Answer from the drawing. Dimensions are ordinates in mm from the lowest x, y and z of the part. Coordinates: 2 decimals unless noted, no trailing zeros. Write each loop counter-clockwise with the first axis right and the second up, starting at its lowest first coordinate (ties: lowest second). Pieces come first, ordered by that corner, then holes.
(1) The part is cut by section B-B on x = 170.5. Determine the outline of the cut face in (y, z), plus the area to 3 significant figures.
(2) The part is cut by section A-A on z = 641. Determine the outline of the cut face in (x, y).
(3) The part is cut by section C-C on x = 481. Determine the outline of the cut face in (y, z).
(4) Straight lines are drawn through the part: line 1 (Z direction, x = 185, y = 15.25); line 2 (Z direction, x = 352.5, y = 16.75); line 3 (X direction, y = 9.25, z = 678.5). For each, find the intervals that lie inside material, in ascending order.
(5) The part is cut by section D-D on y = 7.75. Determine the outline of the cut face in (x, z).
(6) Given P1, Ø5.5, axis at x = 144.5, y = 10, coming from the -Z side, flat-ended and moving along its own axis, determine where the tip first touches the part or whether it passes through.
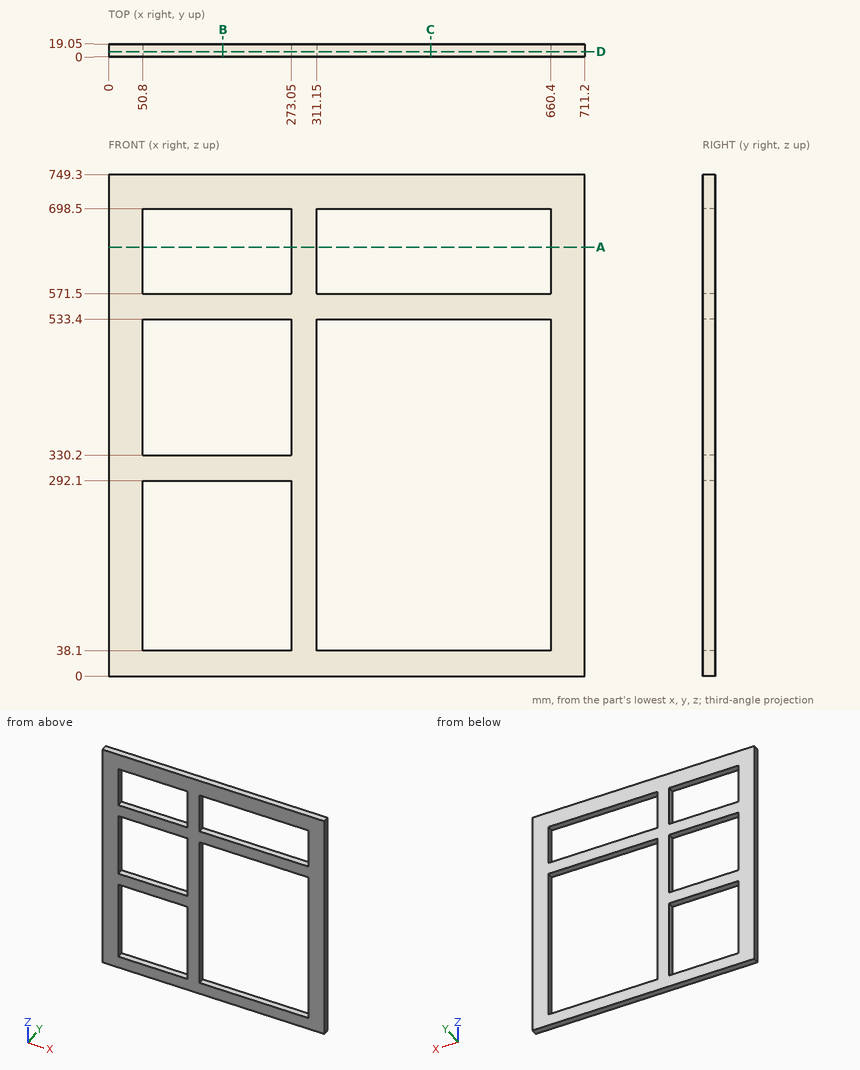
Model answer:
1. outline: (0, 0) - (19.05, 0) - (19.05, 38.1) - (0, 38.1) - close; (0, 292.1) - (19.05, 292.1) - (19.05, 330.2) - (0, 330.2) - close; (0, 533.4) - (19.05, 533.4) - (19.05, 571.5) - (0, 571.5) - close; (0, 698.5) - (19.05, 698.5) - (19.05, 749.3) - (0, 749.3) - close
1. area: 3,150 mm2
2. outline: (0, 0) - (50.8, 0) - (50.8, 19.05) - (0, 19.05) - close; (273.05, 0) - (311.15, 0) - (311.15, 19.05) - (273.05, 19.05) - close; (660.4, 0) - (711.2, 0) - (711.2, 19.05) - (660.4, 19.05) - close
3. outline: (0, 0) - (19.05, 0) - (19.05, 38.1) - (0, 38.1) - close; (0, 533.4) - (19.05, 533.4) - (19.05, 571.5) - (0, 571.5) - close; (0, 698.5) - (19.05, 698.5) - (19.05, 749.3) - (0, 749.3) - close
4. line 1: z = 0 to 38.1, 292.1 to 330.2, 533.4 to 571.5, 698.5 to 749.3
4. line 2: z = 0 to 38.1, 533.4 to 571.5, 698.5 to 749.3
4. line 3: x = 0 to 50.8, 273.05 to 311.15, 660.4 to 711.2
5. outline: (0, 0) - (711.2, 0) - (711.2, 749.3) - (0, 749.3) - close; hole (50.8, 38.1) - (273.05, 38.1) - (273.05, 292.1) - (50.8, 292.1) - close; hole (50.8, 330.2) - (273.05, 330.2) - (273.05, 533.4) - (50.8, 533.4) - close; hole (50.8, 571.5) - (273.05, 571.5) - (273.05, 698.5) - (50.8, 698.5) - close; hole (311.15, 38.1) - (660.4, 38.1) - (660.4, 533.4) - (311.15, 533.4) - close; hole (311.15, 571.5) - (660.4, 571.5) - (660.4, 698.5) - (311.15, 698.5) - close
6. P1: stops at z = 0
